Geometry check sheet. Reference: the model listing, model coordinates, mm. Coordinates: 2 decimals unless noted, no trailing zeros. Order: outer loops, then holes, each group sorted by start corner. A loop starts at its lowest first (then second) coordinate and runs counter-clockwise, first axis right, second up. Notation, with made-up numbers: (22, 82) - (55, 82) arc R22 cw to (55, 98) - close; hole circle Ø7 at (14.5, 20.25). An arc over 180 degrees is marked (long way). Put each result on its own line as item: value.
Autodesk Inventor part; units mm, degrees
ref_plane "YZ Plane" through (0, 0, 0) normal (1, 0, 0) x (0, 1, 0)
ref_plane "XZ Plane" through (0, 0, 0) normal (0, 1, 0) x (-1, 0, 0)
ref_plane "XY Plane" through (0, 0, 0) normal (0, 0, 1) x (1, 0, 0)
sketch "Sketch1" plane through (0, 0, 0) normal (0, 1, 0) x (-1, 0, 0)
  line L0 (0, 0) -> (50.8, 0)
  line L1 (50.8, 0) -> (50.8, -275.4)
  line L2 (50.8, -275.4) -> (0, -275.4)
  line L3 (0, -275.4) -> (0, 0)
  dimension "d0" = 50.8
  dimension "d1" = 275.4
extrude "Extrusion1" add sketch "Sketch1" along normal blind 12.7
sketch "Sketch2" plane through (0, 12.7, 0) normal (0, 1, 0) x (1, 0, 0)
  circle A0 centre (-38.1, 87.7) radius 3.175
  circle A1 centre (-38.1, 187.7) radius 3.175
  line L0 (-50.8, 0) -> (0, 0)
  line L1 (0, 0) -> (0, 275.4)
  dimension "d4" = 87.7
  dimension "d5" = 100
  dimension "d6" = 6.35
  dimension "d7" = 38.1
extrude "Extrusion2" cut sketch "Sketch2" against normal blind 12.7
properties part number "Wood-8"
Q1. Section check B-B on z = -187.7. Record the boundary of the cut face in (x, y) (3 decimals), then the cut area to 3 significant figures.
Answer block:
outline: (-50.8, 0) - (-41.275, 0) - (-41.275, 12.7) - (-50.8, 12.7) - close; (-34.925, 0) - (0, 0) - (0, 12.7) - (-34.925, 12.7) - close
area: 565 mm^2
Q2. Thickness scan on L1, parallel to Z at x = -38.1, y = 7.25 (3 decimals); L2, parallel to X at y = 6.75, z = -87.7 (3 decimals); L3, parallel to Z at x = -36, y = 11. Record the ranges inside material, lowest first. Write a range as [from, to].
Answer block:
L1: z = [-275.4, -190.875], [-184.525, -90.875], [-84.525, 0]
L2: x = [-50.8, -41.275], [-34.925, 0]
L3: z = [-275.4, -190.08], [-185.32, -90.08], [-85.32, 0]
Q3. Section check A-A on x = -38.1. Record the boundary of the cut face in (y, z) (3 decimals).
Answer block:
outline: (0, -275.4) - (12.7, -275.4) - (12.7, -190.875) - (0, -190.875) - close; (0, -184.525) - (12.7, -184.525) - (12.7, -90.875) - (0, -90.875) - close; (0, -84.525) - (12.7, -84.525) - (12.7, 0) - (0, 0) - close
Q4. Draft check along Z on faces 1 (the cylindrical face through (-38.51, 6.44, -190.85)), 2 (the flat face through (-50.8, 6, -136)), 3 (the flat face through (-26, 6, -275.4)). Enter one of: pulls with the +Z half, pulls with the -Z half, needs draft (parallel to the pull), parting line crosses it, or undercut.
Answer block:
face 1: undercut
face 2: needs draft
face 3: pulls with the -Z half
